Autodesk Inventor part; units mm, degrees
ref_plane "YZ Plane" through (0, 0, 0) normal (1, 0, 0) x (0, 1, 0)
ref_plane "XZ Plane" through (0, 0, 0) normal (0, 1, 0) x (-1, 0, 0)
ref_plane "XY Plane" through (0, 0, 0) normal (0, 0, 1) x (1, 0, 0)
sketch "Sketch1" plane through (0, 0, 0) normal (0, 1, 0) x (-1, 0, 0)
  line L0 (-59.5, 59.5) -> (59.5, 59.5)
  line L1 (59.5, 59.5) -> (59.5, -59.5)
  line L2 (59.5, -59.5) -> (-59.5, -59.5)
  line L3 (-59.5, -59.5) -> (-59.5, 59.5)
  line L4 (-59.5, 59.5) -> (59.5, -59.5) construction
  line L5 (59.5, 59.5) -> (-59.5, -59.5) construction
  circle A0 centre (52.4, 52.4) radius 1.5
  circle A1 centre (52.4, -52.4) radius 1.5
  arc A2 (58, 23.2863) -> (23.2863, 58) centre (0, 0) ccw
  arc A3 (23.2863, -58) -> (58, -23.2863) centre (0, 0) ccw
  arc A4 (-58, -23.2863) -> (-23.2863, -58) centre (0, 0) ccw
  arc A5 (-23.2863, 58) -> (-58, 23.2863) centre (0, 0) ccw
  line L6 (23.2863, 58) -> (-23.2863, 58)
  line L7 (-58, 23.2863) -> (-58, -23.2863)
  line L8 (-23.2863, -58) -> (23.2863, -58)
  line L9 (58, -23.2863) -> (58, 23.2863)
  arc A6 (59.5, 52.4) -> (52.4, 59.5) centre (52.4, 52.4) ccw
  line L10 (48.2954, 59.5) -> (44.1942, 44.1942)
  line L11 (44.1942, 44.1942) -> (59.5, 48.2954)
  circle A7 centre (0, 0) radius 28
  circle A8 centre (0, 0) radius 29.5
  line L12 (44.7213, 43.6607) -> (21.3832, 20.3226)
  line L13 (20.3226, 21.3832) -> (43.6607, 44.7213)
  circle A9 centre (0, 0) radius 43.6607 construction
  line L14 (44.7213, 43.6607) -> (0, 43.6607) construction
  circle A10 centre (0, 0) radius 44.4107
  circle A11 centre (0, 0) radius 42.9107
  point P0 (0, 58)
  dimension "d0" = 119
  dimension "d1" = 3
  dimension "d2" = 104.8
  dimension "d4" = 62.5
  dimension "d7" = 116
  dimension "d9" = 30
  dimension "d38" = 56
  dimension "d39" = 1.5
  dimension "d40" = 1.5
  dimension "d41" = 1.5
  dimension "d83" = 1.5
  dimension "d84" = 0.75
extrude "Extrusion8" add sketch "Sketch1" along normal blind 3.175 contours L0 L10 L11 L1 L2 L3 | L0 A6 L1 L11 L10 | L0 L1 A6 | A8 | A0 | A1
extrude "Extrusion9" add sketch "Sketch1" along normal blind 3.175 contours A2 L12 A10 L13 | L12 A11 L13 A10 | L12 A8 L13 A11 picked at (31.1052, 30.2803) picked at (23.6041, 24.429)
extrude "Extrusion10" cut sketch "Sketch1" along normal up to next contours L0 L1 A6 | A0
pattern_circular "Circular Pattern4" count 4 over 360 about axis through (0, 0, 0) along (0, 1, 0) of "Extrusion10", "Extrusion9"
sketch "Sketch4" plane through (0, 0, 0) normal (0, -1, 0) x (1, 0, 0)
  arc A0 (-52.4, 59.5) -> (-59.5, 52.4) centre (-52.4, 52.4) ccw
  line L0 (-52.4, 59.5) -> (52.4, 59.5)
  line L1 (-59.5, -52.4) -> (-59.5, 52.4)
  arc A1 (-59.5, -52.4) -> (-52.4, -59.5) centre (-52.4, -52.4) ccw
  line L2 (52.4, -59.5) -> (-52.4, -59.5)
  arc A2 (52.4, -59.5) -> (59.5, -52.4) centre (52.4, -52.4) ccw
  line L3 (59.5, 52.4) -> (59.5, -52.4)
  arc A3 (59.5, 52.4) -> (52.4, 59.5) centre (52.4, 52.4) ccw
  line L4 (52.4, 58) -> (-52.4, 58)
  arc A4 (-52.4, 58) -> (-58, 52.4) centre (-52.4, 52.4) ccw
  line L5 (-58, 52.4) -> (-58, -52.4)
  arc A5 (-58, -52.4) -> (-52.4, -58) centre (-52.4, -52.4) ccw
  line L6 (-52.4, -58) -> (52.4, -58)
  arc A6 (52.4, -58) -> (58, -52.4) centre (52.4, -52.4) ccw
  line L7 (58, -52.4) -> (58, 52.4)
  arc A7 (58, 52.4) -> (52.4, 58) centre (52.4, 52.4) ccw
  line L8 (-58, 38.8804) -> (-38.8804, 58)
  line L9 (-52.4, 52.4) -> (-48.4402, 48.4402) construction
  line L10 (-52.4, 52.4) -> (-56.3598, 56.3598) construction
  circle A8 centre (-52.4, 52.4) radius 1.5
  point P0 (0, 0)
  dimension "d51" = 1.5
  dimension "d52" = 45
extrude "Extrusion11" add sketch "Sketch4" along normal blind 22.225 contours L0 A3 L3 A2 L2 A1 L1 A0
extrude "Extrusion12" add sketch "Sketch4" along normal blind 19.05 contours L8 L5 A4 L4
pattern_circular "Circular Pattern5" count 4 over 360 about axis through (0, 0, 0) along (0, 1, 0) of "Extrusion12"
extrude "Extrusion18" add sketch "Sketch1" along normal blind 3.175 contours A10 L13 A11 L12 | L12 A11 L13 A10
equation "\"d0\" = length"
equation "\"d1\" = holeSize"
equation "\"d2\" = dHoles"
equation "\"d4\" = 0.5 * fanDia"
equation "\"d7\" = fanCutOff"
equation "\"d38\" = fanCenter"
equation "\"d40\" = d39"
equation "\"d41\" = d40"
equation "\"d83\" = d39"
equation "\"d84\" = 0.5 * d39"
equation "\"d51\" = d40"
equation "\"d55\" = filterHeight"
equation "\"holeSize\" = 3"
equation "\"filterHeight\" = 19.05"
properties part number "filterFrame"
Geometry check sheet. Reference: the model listing, model coordinates, mm. A direction names the side the tool comes from. Coordinates: 2 decimals unless noted, no trailing zeros. Loops run counter-clockwise (first coordinate to the right, second up) from the corner with the lowest first, then second, coordinate; pieces in that order, holes last. Notation, with made-up numbers: (64, 54.25) - (92, 54.25) arc R21 ccw to (92, 83.25) - close; hole circle Ø5 at (85, 41). An arc over 180 degrees is marked (long way). Use one line per item in the form item = value. Start each with the question number.
Item 1: Thickness scan on probe 1 along Z at (x, y) = (-9.5, -9); probe 2 along Z at (x, y) = (52.4, 0.9). Record the ranges inside material, lowest first.
Item 2: Tool access check on faces 1 (the face through (-1, -9, 59.5)), 2 (the face through (-25, 1.57, 26.06)), 3 (the face through (-56.32, -20.62, -56.4)). Record the directions out of +Z, -Z, +X, -X, +Y, -Y that give a thin tool (end or side, any length) a straight path to the whole face; none if there is none.
Item 3: Gauge pin test, flat end, axial feed: pin 1 (4 mm diameter, centred on x = -52.4, z = -52.4, fed in from -Y). Record the tip position at first contact, or that the pin passes through.
Item 4: Mould release check, pull along X, two halves, no side actions. Record for faces 4 (the face through (1, -9, -59.5)), 5 (the face through (25.13, 1.57, 26.19)), 6 (the face through (-51, -19.05, 51)): +X half, -X half, draft (parallel to the pull), parting line (faces both ways), or undercut.
Item 5: Section check A-A, the plane y = -2.5. Enter the section's corners in (x, z).
Item 6: Section check C-C, the plane x = -8. Enter the section's corners in (y, z) (3 decimals), and give its area (3 significant figures).
Item 7: Section check B-B, the plane z = -6. Enter the section's corners in (x, y) (3 decimals).
Computed:
q1.probe_1 = -59.5 to -58, 58 to 59.5
q1.probe_2 = -59.5 to -53.9, -50.9 to -34.07, 34.07 to 50.9, 53.9 to 59.5
q2.face_1 = +Z, +X, -X, +Y, -Y
q2.face_2 = +Y, -Y
q2.face_3 = -Y
q3.pin_1 = -19.05
q4.face_4 = draft
q4.face_5 = undercut
q4.face_6 = undercut
q5.outline = (-59.5, -52.4) arc R7.1 ccw to (-52.4, -59.5) - (52.4, -59.5) arc R7.1 ccw to (59.5, -52.4) - (59.5, 52.4) arc R7.1 ccw to (52.4, 59.5) - (-52.4, 59.5) arc R7.1 ccw to (-59.5, 52.4) - close; hole (-58, -38.88) - (-38.88, -58) - (38.88, -58) - (58, -38.88) - (58, 38.88) - (38.88, 58) - (-38.88, 58) - (-58, 38.88) - close; hole circle Ø3 at (-52.4, -52.4); hole circle Ø3 at (-52.4, 52.4); hole circle Ø3 at (52.4, -52.4); hole circle Ø3 at (52.4, 52.4)
q6.outline = (-22.225, -59.5) - (3.175, -59.5) - (3.175, -58) - (-22.225, -58) - close; (-22.225, 58) - (3.175, 58) - (3.175, 59.5) - (-22.225, 59.5) - close; (0, -43.684) - (3.175, -43.684) - (3.175, -42.158) - (0, -42.158) - close; (0, -28.395) - (3.175, -28.395) - (3.175, -26.833) - (0, -26.833) - close; (0, 26.833) - (3.175, 26.833) - (3.175, 28.395) - (0, 28.395) - close; (0, 42.158) - (3.175, 42.158) - (3.175, 43.684) - (0, 43.684) - close
q6.area = 95.8 mm2
q7.outline = (-59.5, -22.225) - (-58, -22.225) - (-58, 3.175) - (-59.5, 3.175) - close; (-44.004, 0) - (-42.489, 0) - (-42.489, 3.175) - (-44.004, 3.175) - close; (-28.883, 0) - (-27.35, 0) - (-27.35, 3.175) - (-28.883, 3.175) - close; (27.35, 0) - (28.883, 0) - (28.883, 3.175) - (27.35, 3.175) - close; (42.489, 0) - (44.004, 0) - (44.004, 3.175) - (42.489, 3.175) - close; (58, -22.225) - (59.5, -22.225) - (59.5, 3.175) - (58, 3.175) - close
